```python
from build123d import *

# Parameters (mm, degrees)
SKETCH_R           = 10
PAD_DEPTH          = 15
POCKET_DEPTH       = 2
SKETCH002_R        = 1.75
POCKET001_DEPTH    = 15.001
POCKET002_DEPTH    = 79.032242
POLARPATTERN_COUNT = 20


with BuildPart() as part:
    # Sketch → Pad (new body)
    with BuildSketch(Plane.XY):
        Circle(SKETCH_R)
    extrude(amount=PAD_DEPTH)

    # Sketch001 → Pocket (cut)
    with BuildSketch(Plane.XY.offset(3)):
        Polygon((4.618802, 0), (2.309401, 4), (-2.309401, 4), (-4.618802, 0), (-2.309401, -4), (2.309401, -4), align=None)
    extrude(amount=POCKET_DEPTH, mode=Mode.SUBTRACT)

    # Sketch002 → Pocket001 (cut, through all)
    with BuildSketch(Plane.XY):
        Circle(SKETCH002_R)
    extrude(amount=POCKET001_DEPTH, mode=Mode.SUBTRACT)

    # Sketch003 → Pocket002 (cut, through all)
    with BuildSketch(Plane.XY):
        Polygon((-0.206247, 10.247925), (0.206247, 10.247925), (0, 9.75), align=None)
    pocket002 = extrude(amount=POCKET002_DEPTH, mode=Mode.SUBTRACT)

    # PolarPattern: Pocket002 ×20 about axis
    polarpattern_axis = Axis((0, 0, 0), (0, 0, 1))
    for i in range(1, POLARPATTERN_COUNT):
        add(pocket002.rotate(polarpattern_axis, i * 360 / POLARPATTERN_COUNT), mode=Mode.SUBTRACT)


solid = part.part
```
Can you work these out from the model? Positions are in its coordinate system, mm. A direction names the side the tool comes from. Coordinates: 2 decimals unless noted, no trailing zeros. Order: outer loops, then holes, each group sorted by start corner. A loop starts at its lowest first (then second) coordinate and runs counter-clockwise, first axis right, second up.
1. I need wall thicknesses on line 1 (Y direction, x = -1, z = 9.5); line 2 (Y direction, x = 1.5, z = 7.75); line 3 (X direction, y = 0.5, z = 2.5). Which ranges of each line are inside material? Lowest first, please.
2. I'm going to push flat-ended pins straight in: pin 1 (4 mm diameter, centred on x = 4, y = 6.5, fed in from -Z); pin 2 (0.6 mm diameter, centred on x = 0.5, z = 4.5, fed in from +Y); pin 3 (3 mm diameter, centred on x = 0, y = 0, fed in from +Z); pin 4 (5 mm diameter, centred on x = -7.5, z = 6.5, fed in from -Y). Where does each tip first touch, or does it pass through?
3. If we section it at A-A (y = 8.75): Please give me the cut outline in (x, z), then the cut area to 3 significant figures.
4. If we section it at B-B (x = -8.5): Please give me the cut outline in (y, z).
5. Thinking about a two-plate mould opening in X: for faces 3 (the face through (1.617, -0.67, 9.93)), 4 (the face through (-1.585, -9.874, 7.395)), 5 (the face through (-3.448, 2.028, 3.986)), 6 (the face through (1.585, 9.874, 7.395)), which applies, +X half, -X half, draft (parallel to the pull), parting line (faces both ways), or undercut?
6. For faces 1 (the face through (3.448, -2.028, 3.986)), 2 (the face through (-1.54, 9.88, 7.4)), which set-ups out of +Z, -Z, +X, -X, +Y, -Y let a thin tool reach every point of the face, with its end or its side?
Entries:
1. line 1: y = -9.95 to -1.44, 1.44 to 9.95
1. line 2: y = -9.89 to -0.9, 0.9 to 9.89
1. line 3: x = -9.99 to -1.68, 1.68 to 9.99
2. pin 1: stops at z = 0
2. pin 2: stops at y = 10
2. pin 3: passes through
2. pin 4: stops at y = -8.66
3. outline: (-4.84, 0) - (4.84, 0) - (4.84, 15) - (-4.84, 15) - close
3. area: 145 mm2
4. outline: (-5.27, 0) - (5.27, 0) - (5.27, 15) - (-5.27, 15) - close
5. face 3: undercut
5. face 4: -X half
5. face 5: undercut
5. face 6: +X half
6. face 1: none
6. face 2: +Z, -Z, -X, +Y
